Geometry check sheet. Reference: the model listing, model coordinates, mm. A direction names the side the tool comes from. Round coordinates to 2 decimals unless told otherwise and drop trailing zeros. Order: outer loops, then holes, each group sorted by start corner. A loop starts at its lowest first (then second) coordinate and runs counter-clockwise, first axis right, second up.
```python
from build123d import *

# Parameters (mm, degrees)
F1_DEPTH = 82.55
F2_R     = 76.2


with BuildPart() as f1:
    # F0 (on Front) → F1 (new body, symmetric)
    with BuildSketch(Plane.XZ):
        Polygon((161.29, -508), (161.29, 508), (115.3964, 508), (115.3964, 190.5), (0, 190.5), (-113.2036, 190.5), (-113.2036, 508), (-161.29, 508), (-161.29, -508), (-115.3964, -508), (-115.3964, -190.5), (0, -190.5), (113.2036, -190.5), (113.2036, -508), align=None)
    extrude(amount=F1_DEPTH, both=True)

    # F2
    f2_edges = [f1.edges().sort_by_distance(p)[0] for p in [
        (1.0964, -82.55, 190.5),
        (1.0964, 82.55, 190.5),
        (-1.0964, 82.55, -190.5),
        (-1.0964, -82.55, -190.5),
    ]]
    fillet(f2_edges, radius=F2_R)


solid = f1.part
```
(1) Depth check by flat-ended pin: P1, Ø8, axis at x = -47.5, y = 18, coming from the +Z side (3 decimals); P2, Ø1, axis at x = -94, y = 64, coming from the -Z side; P3, Ø6, axis at x = 25.5, z = -168.5, coming from the +Y side. Enter the tip coordinate at first touch or a pass-through.
Returned:
P1: stops at z = 190.115
P2: stops at z = -164.7
P3: stops at y = 62.79
(2) Sectioned sample at A-A, the plane x = -79.5. Record the cut outline in (y, z).
Returned:
outline: (-82.55, -114.3) arc R76.2 ccw to (-6.35, -190.5) - (6.35, -190.5) arc R76.2 ccw to (82.55, -114.3) - (82.55, 114.3) arc R76.2 ccw to (6.35, 190.5) - (-6.35, 190.5) arc R76.2 ccw to (-82.55, 114.3) - close
(3) Material ranges on line 1 (X direction, y = 18, z = -331); line 2 (X direction, y = 55, z = 192); line 3 (Z direction, x = -22, y = -10.5), recorded low to high.
Returned:
line 1: x = -161.29 to -115.4, 113.2 to 161.29
line 2: x = -161.29 to -113.2, 115.4 to 161.29
line 3: z = -190.39 to 190.39
(4) Draft check along X on faces 1 (the flat face through (139, -1, 508)), 2 (the flat face through (161.29, -1, -7)), 3 (the cylindrical face through (0.504, 59.636, -168.771)). Enter one of: released by +X, released by -X, zero draft, split by the parting line, or undercut.
Returned:
face 1: zero draft
face 2: released by +X
face 3: undercut
(5) Sectioned sample at D-D, the plane z = 156.5. Record the cut outline in (x, y), and give its area (3 significant figures).
Returned:
outline: (-161.29, -82.55) - (-113.2, -82.55) - (-113.2, -69.8) - (115.4, -69.8) - (115.4, -82.55) - (161.29, -82.55) - (161.29, 82.55) - (115.4, 82.55) - (115.4, 69.8) - (-113.2, 69.8) - (-113.2, 82.55) - (-161.29, 82.55) - close
area: 47,400 mm2
(6) Sectioned sample at C-C, the plane y = -23. Record the cut outline in (x, z).
Returned:
outline: (-161.29, -508) - (-115.4, -508) - (-115.4, -188.66) - (113.2, -188.66) - (113.2, -508) - (161.29, -508) - (161.29, 508) - (115.4, 508) - (115.4, 188.66) - (-113.2, 188.66) - (-113.2, 508) - (-161.29, 508) - close
(7) Sectioned sample at B-B, the plane z = -420.5. Record the cut outline in (x, y).
Returned:
outline: (-161.29, -82.55) - (-115.4, -82.55) - (-115.4, 82.55) - (-161.29, 82.55) - close; (113.2, -82.55) - (161.29, -82.55) - (161.29, 82.55) - (113.2, 82.55) - close
(8) Set-up check for faces 4 (the cylindrical face through (-0.504, 59.636, 168.771)), 5 (the cylindrical face through (-0.504, -59.636, 168.771)), 6 (the flat face through (-161.29, -1, 7)), 7 (the cylindrical face through (0.504, -59.636, -168.771)): record each of +Z, -Z, +X, -X, +Y, -Y from which the full face is reachable in a straight line by a thin tool's end or side.
Returned:
face 4: +Z, +Y
face 5: +Z, -Y
face 6: +Z, -Z, -X, +Y, -Y
face 7: -Z, -Y
